Autodesk Inventor part; units mm, degrees
ref_plane "Arbeitsebene1" through (0, 0, 0) normal (0, 0, 1) x (1, 0, 0)
ref_plane "YZ Plane" through (0, 0, 0) normal (1, 0, 0) x (0, 1, 0)
ref_plane "XZ Plane" through (0, 0, 0) normal (0, 1, 0) x (-1, 0, 0)
sketch "Skizze1" plane through (0, 0, 0) normal (0, 0, 1) x (1, 0, 0)
  line L0 (0, 0) -> (0, 95)
  line L1 (0, 95) -> (52.5, 95)
  line L2 (52.5, 95) -> (70, 78.185) construction
  line L3 (70, 78.185) -> (100, 54.4042) construction
  line L4 (100, 54.4042) -> (60, 22.4311) construction
  line L5 (60, 22.4311) -> (26.3149, 0) construction
  spline S0 degree 4 poles (52.5, 95) (70, 78.185) (100, 54.4042) (60, 22.4311) (26.3149, 0) knots 1 1 1 1 1 2 2 2 2 2
  line L6 (0, 0) -> (26.3149, 0)
  dimension "d0" = 95
  dimension "d12" = 105
  dimension "d13" = 200
  dimension "d14" = 140
  dimension "d15" = 120
  dimension "d16" = 16.815
  dimension "d17" = 40.5958
  dimension "d18" = 72.5689
  dimension "d20" = 52.6298
revolve "Umdrehung1" add sketch "Skizze1" angle 360 about axis through (0, 0, 0) along (0, 1, 0)
shell "Wandung1" thickness 1 removed faces 1 at (15.8747, 95, 30.7926)
ref_plane "Arbeitsebene1" through (0, 0, 0) normal (0, 0, 1) x (1, 0, 0)
sketch "Skizze3" plane through (0, 0, 0) normal (0, 0, 1) x (1, 0, 0)
  line L0 (26.3149, 0) -> (-26.3149, 0)
  line L1 (52.5, 95) -> (-52.5, 95)
  line L2 (51.0567, 95) -> (-51.0567, 95)
  line L3 (26.0122, 1) -> (-26.0122, 1)
  arc A0 (-9, -27.1862) -> (-26.3149, 0) centre (-39, -27.1862) ccw
  line L4 (0, 0) -> (0, -105)
  line L5 (-9, -27.1862) -> (-9, -75.1862)
  arc A1 (0, -103.1862) -> (-14.9609, -107.1862) centre (0, -133.1648) ccw
  line L6 (-14.9609, -107.1862) -> (-37.5, -107.1862)
  line L7 (-37.5, -107.1862) -> (-37.5, -103.6862)
  arc A2 (-37.5, -103.6862) -> (-9, -75.1862) centre (-37.5, -75.1862) ccw
  point P0 (-37.5, -105.4362)
  point P1 (0, -52.5)
  dimension "d24" = 200
  dimension "d25" = 30
  dimension "d26" = 80
  dimension "d27" = 75
  dimension "d28" = 4
  dimension "d30" = 9
  dimension "d32" = 29.9218
  dimension "d33" = 3.5
revolve "Umdrehung2" add sketch "Skizze3" angle 360 about axis through (0, 0, 0) along (0, -1, 0)
properties part number "Glas" material "Glas"
Input: part model. Units: mm. Frame: model coordinates. Round coordinates to 2 decimals unless told otherwise and drop trailing zeros. Order: outer loops, then holes, each group sorted by start corner. A loop starts at its lowest first (then second) coordinate and runs counter-clockwise, first axis right, second up. Notation, with made-up numbers: (24.5, 14) - (51.5, 14) arc R19 ccw to (51.5, 41) - close; hole circle Ø2 at (-37, 66). An arc over 180 degrees is marked (long way). Answer in a Markdown table with one row per item.
Item 1: Mould query, pull axis Y, two halves, no side actions, for faces 1 (the cylindrical face through (1.172, -51.522, -8.923)), 2 (the cylindrical face through (4.88, -105.41, 37.18)), 3 (the flat face through (1, -107.186, 16)), 4 (the flat face through (11.4, 95, 50.3)). Classes: released by +Y, released by -Y, zero draft, split by the parting line, or undercut.
Model answer:
| item | result |
|---|---|
| face 1 | undercut |
| face 2 | zero draft |
| face 3 | released by -Y |
| face 4 | released by +Y |
Item 2: Section query B-B (y = -86.5). Return the cut outline in (x, z), then the cut area to 3 significant figures.
Model answer:
| item | result |
|---|---|
| outline | circle Ø22.68 at (0, 0) |
| area | 404 mm² |
Item 3: Pin query (flat end, axial travel): pin 1 (10 mm diameter, centred on x = 8.5, y = -71, fed in from +Z); pin 2 (1 mm diameter, centred on y = 65.5, z = 21.5, fed in from +X); pin 3 (3 mm diameter, centred on x = -17.5, z = -36.5, fed in from +Y); pin 4 (5 mm diameter, centred on x = -42.5, z = -27.5, fed in from +Y). Return the tip coordinate at first contact, or that it passes through.
Model answer:
| item | result |
|---|---|
| pin 1 | stops at z = 8.29 |
| pin 2 | stops at x = 71.72 |
| pin 3 | stops at y = 12.31 |
| pin 4 | stops at y = 95 |
Item 4: Section query A-A (y = -65.5). Return the cut outline in (x, z).
Model answer:
| item | result |
|---|---|
| outline | circle Ø18 at (0, 0) |
Item 5: Line query: line 1 (Y direction, x = 54, z = 1.5); line 2 (X direction, y = 62, z = 56.5) (3 decimals); line 3 (Y direction, x = -29.5, z = -18.5). Output: solid intervals per line, ascending.
Model answer:
| item | result |
|---|---|
| line 1 | y = 20.98 to 22.34, 92.17 to 93.55 |
| line 2 | x = -49.914 to -48.375, 48.375 to 49.914 |
| line 3 | y = -107.19 to -103.56, 5.82 to 7.05 |
